```python
from build123d import *

# Parameters (mm, degrees)
F1_DEPTH  = 130
F2_R      = 4.5
F2_R_2    = 17.4
F2_R_3    = 3.25
F3_DEPTH  = 4
F1_FACE_W = 50
F1_FACE_H = 130
F5_DEPTH  = 25.001
F7_R      = 12.5
F8_DEPTH  = 50.001
F7_R_2    = 3.25
F9_DEPTH  = 50.001


with BuildPart() as f1:
    # F0 (on Front) → F1 (new body)
    with BuildSketch(Plane.XZ):
        Polygon((25, -25), (25, 25), (22, 25), (22, -22), (-22, -22), (-22, 25), (-25, 25), (-25, -25), align=None)
    extrude(amount=F1_DEPTH)

    # F2 (on Front) → F3 (join)
    with BuildSketch(Plane.XZ):
        with BuildLine():
            Line((-22, 25), (-22, -22))
            Line((-22, -22), (22, -22))
            Line((22, -22), (22, 68))
            Line((22, 68), (10.0712478979, 68))
            ThreePointArc((10.0712478979, 68), (0, 57.9287521021), (-10.0712478979, 68))
            Line((-10.0712478979, 68), (-22, 68))
            Line((-22, 68), (-22, 25))
        make_face()
        with Locations((0, -12.6673281193)):
            Circle(F2_R, mode=Mode.SUBTRACT)
        with Locations((0, 15.7326718807)):
            Circle(F2_R_2, mode=Mode.SUBTRACT)
        with Locations((-16, 62)):
            Circle(F2_R_3, mode=Mode.SUBTRACT)
        with Locations((0, 44.3326718807)):
            Circle(F2_R, mode=Mode.SUBTRACT)
        with Locations((16, 62)):
            Circle(F2_R_3, mode=Mode.SUBTRACT)
    extrude(amount=F3_DEPTH)

    # F4 (on Top) + F1_face (on face) → F5 (cut, through all)
    with BuildSketch(Plane.XY):
        with BuildLine():
            Line((-12.9999999838, -48.7308816649), (-12.9972082527, -104.5789601389))
            ThreePointArc((-12.9972082527, -104.5789601389), (-0.1347084156, -117.8476645499), (13, -104.8483625054))
            Line((13, -104.8483625054), (13, -48.7302318215))
            ThreePointArc((13, -48.7302318215), (-0.0003249217, -35.7302318256), (-12.9999999838, -48.7308816649))
        make_face()
        with BuildLine():
            Line((9.9999410594, -5.0000000003), (-9.9515041286, -5.0002351905))
            ThreePointArc((-9.9515041286, -5.0002351905), (-14.9977215138, -9.8490706455), (-10.2532994666, -14.9935798161))
            Line((-10.2532994666, -14.9935798161), (-9.7498665822, -14.9937394078))
            Line((-9.7498665822, -14.9937394078), (9.9984149657, -14.9999997488))
            ThreePointArc((9.9984149657, -14.9999997488), (14.9999999418, -10.0007630468), (9.9999410594, -5.0000000003))
        make_face()
        with BuildLine():
            Line((-9.7498665822, -14.9937394078), (-10.2532994666, -14.9935798161))
            ThreePointArc((-10.2532994666, -14.9935798161), (-10.0015850343, -14.9999997488), (-9.7498665822, -14.9937394078))
        make_face()
    with BuildSketch(Plane(origin=(0, -65, -25), x_dir=(1, 0, 0), z_dir=(0, 0, -1))):
        Rectangle(F1_FACE_W, F1_FACE_H)
    extrude(amount=-F5_DEPTH, dir=(0, 0, 1), mode=Mode.SUBTRACT)

    # F7 (on face) → F8 (cut, through all)
    with BuildSketch(Plane(origin=(-25, 0, 0), x_dir=(0, -1, 0), z_dir=(-1, 0, 0))):
        with Locations((31.6511541605, 0)):
            Circle(F7_R)
        with Locations((92.5872474909, 0)):
            Circle(F7_R)
    extrude(amount=-F8_DEPTH, mode=Mode.SUBTRACT)

    # F7 (on face) → F9 (cut, through all)
    with BuildSketch(Plane(origin=(-25, 0, 0), x_dir=(0, -1, 0), z_dir=(-1, 0, 0))):
        with Locations((92.5872474909, 0)):
            Circle(F7_R)
        with Locations((31.6511541605, 0)):
            Circle(F7_R)
        with Locations((92.3290103674, 19)):
            Circle(F7_R_2)
        with Locations((82.3290103674, 19)):
            Circle(F7_R_2)
        with Locations((72.3290103674, 19)):
            Circle(F7_R_2)
        with Locations((62.3290103674, 19)):
            Circle(F7_R_2)
        with Locations((52.3290103674, 19)):
            Circle(F7_R_2)
        with Locations((42.3290103674, 19)):
            Circle(F7_R_2)
    extrude(amount=-F9_DEPTH, mode=Mode.SUBTRACT)


solid = f1.part
```
The model under review builds one solid part; all positions refer to its coordinate system, in mm. A direction names the side the tool comes from. Round coordinates to 2 decimals unless told otherwise and drop trailing zeros. Loops run counter-clockwise (first coordinate to the right, second up) from the corner with the lowest first, then second, coordinate; pieces in that order, holes last. Notation, with made-up numbers: (-4.75, 89) -> (44.25, 89) arc R34 cw to (44.25, 127) -> close; hole circle Ø2 at (33, -4). An arc over 180 degrees is marked (long way). Answer as a JSON object with one key per item and string values. Group by question number.
1) We need section A-A on x = 0. Write out the cut boundary in (y, z), then the cut area to 3 significant figures.
2) For pin 1 Ø12 at (x, z) = (16, 1) entering from +Y; pin 2 Ø3 at (x, z) = (4.5, 49) entering from -Y; pin 3 Ø4 at (y, z) = (-62.33, 19) entering from -X; pin 4 Ø8 at (x, y) = (-17, -110.5) entering from +Z, all flat-tipped, find the tip position at first contact; note any pin that passes through.
3) For faces 4 (the face through (-3.772, -1.972, -1.254)), 5 (the face through (13, -77, -23)), list the 3-axis set-ups (+Z, -Z, +X, -X, +Y, -Y) from which the entire face can be reached by the end or side of a thin tool; tool diameter is ignored.
4) For line 1 (Z direction, x = 0, y = -1.3); line 2 (Z direction, x = 23, y = -90); line 3 (Y direction, x = 19.5, z = 23), list the stretches that pass through material, from the lowest coordinate up. Write a range as [from, to].
5) We need section B-B on y = -98. Write out the cut boundary in (x, z).
6) Mouldability with a two-part tool opening along Y and no side actions: class faces 1 (the face through (22, -66, 2)), 2 (the face through (0, -4, 34)), 3 (the face through (-23.52, -104.51, 3.75)) as released by +Y, released by -Y, zero draft, split by the parting line, or undercut.
7) We need section D-D on y = -21. Write out the cut boundary in (x, z).
8) We need section C-C on z = 0. Write out the cut boundary in (x, y), then the cut area to 3 significant figures.
Result set:
{
 "1": {"outline": "(-130, -25) -> (-117.85, -25) -> (-117.85, -22) -> (-130, -22) -> close; (-35.73, -25) -> (-15, -25) -> (-15, -22) -> (-35.73, -22) -> close; (-5, -25) -> (0, -25) -> (0, -17.17) -> (-4, -17.17) -> (-4, -22) -> (-5, -22) -> close; (-4, -8.17) -> (0, -8.17) -> (0, -1.67) -> (-4, -1.67) -> close; (-4, 33.13) -> (0, 33.13) -> (0, 39.83) -> (-4, 39.83) -> close; (-4, 48.83) -> (0, 48.83) -> (0, 57.93) -> (-4, 57.93) -> close", "area": "222 mm²"},
 "2": {"pin 1": "y = 0", "pin 2": "y = -4", "pin 3": "through", "pin 4": "z = -22"},
 "3": {"face 4": "+Y, -Y", "face 5": "+Z, -Z"},
 "4": {"line 1": "[-25, -17.17], [-8.17, -1.67], [33.13, 39.83], [48.83, 57.93]", "line 2": "[-25, -12.23], [12.23, 16.73], [21.27, 25]", "line 3": "[-4, 0]"},
 "5": {"outline": "(-25, -25) -> (-13, -25) -> (-13, -22) -> (-22, -22) -> (-22, -11.27) -> (-25, -11.27) -> close; (-25, 11.27) -> (-22, 11.27) -> (-22, 25) -> (-25, 25) -> close; (13, -25) -> (25, -25) -> (25, -11.27) -> (22, -11.27) -> (22, -22) -> (13, -22) -> close; (22, 11.27) -> (25, 11.27) -> (25, 25) -> (22, 25) -> close"},
 "6": {"face 1": "zero draft", "face 2": "released by -Y", "face 3": "undercut"},
 "7": {"outline": "(-25, -25) -> (25, -25) -> (25, -6.54) -> (22, -6.54) -> (22, -22) -> (-22, -22) -> (-22, -6.54) -> (-25, -6.54) -> close; (-25, 6.54) -> (-22, 6.54) -> (-22, 25) -> (-25, 25) -> close; (22, 6.54) -> (25, 6.54) -> (25, 25) -> (22, 25) -> close"},
 "8": {"outline": "(-25, -130) -> (-22, -130) -> (-22, -105.09) -> (-25, -105.09) -> close; (-25, -80.09) -> (-22, -80.09) -> (-22, -44.15) -> (-25, -44.15) -> close; (-25, -19.15) -> (-22, -19.15) -> (-22, -4) -> (-7.43, -4) -> (-7.43, 0) -> (-25, 0) -> close; (7.43, -4) -> (22, -4) -> (22, -19.15) -> (25, -19.15) -> (25, 0) -> (7.43, 0) -> close; (22, -130) -> (25, -130) -> (25, -105.09) -> (22, -105.09) -> close; (22, -80.09) -> (25, -80.09) -> (25, -44.15) -> (22, -44.15) -> close", "area": "597 mm²"}
}
